Build history of the part. All positions in model axes, mm. Round coordinates to 2 decimals unless told otherwise and drop trailing zeros. Loops run counter-clockwise (first coordinate to the right, second up) from the corner with the lowest first, then second, coordinate; pieces in that order, holes last.
from build123d import *

# Parameters (mm, degrees)
EXTRUDE1_DEPTH = 25


with BuildPart() as part:
    # Sketch1 → Extrude1 (new body, symmetric)
    with BuildSketch(Plane.XY):
        with BuildLine():
            Line((0, -3), (0, -53.784988575))
            Line((0, -53.784988575), (0, -108))
            ThreePointArc((0, -108), (1.951109669, -110.810663458), (5.266552715, -109.96538515))
            ThreePointArc((5.266552715, -109.96538515), (8.33076313, -107.102662764), (11.924538917, -104.941797077))
            Line((11.924538917, -104.941797077), (78.267854785, -74.00540082))
            ThreePointArc((78.267854785, -74.00540082), (79.819077862, -72.312537889), (79.718923361, -70.018622673))
            Line((79.718923361, -70.018622673), (77.733454722, -65.760771437))
            ThreePointArc((77.733454722, -65.760771437), (76.399777201, -64.367593723), (74.493586828, -64.074202964))
            Line((74.493586828, -64.074202964), (49.961112633, -68.399940068))
            ThreePointArc((49.961112633, -68.399940068), (35.016620352, -65.086825893), (26.791994019, -52.176748561))
            Line((26.791994019, -52.176748561), (22.477002989, -27.705218377))
            ThreePointArc((22.477002989, -27.705218377), (21.821246743, -25.05746196), (20.811309078, -22.523560578))
            Line((20.811309078, -22.523560578), (10.816867263, -1.701806797))
            ThreePointArc((10.816867263, -1.701806797), (9.710018402, -0.460848606), (8.11229809, 0))
            Line((8.11229809, 0), (3, 0))
            ThreePointArc((3, 0), (0.878679656, -0.878679656), (0, -3))
        make_face()
    extrude(amount=EXTRUDE1_DEPTH, both=True)


solid = part.part
(1) Slice it at A-A on z = 13. List the corners of the cut face in (x, y), plus the area to 3 significant figures.
Responses:
outline: (0, -108) arc R3 ccw to (5.27, -109.97) arc R20 cw to (11.92, -104.94) - (78.27, -74.01) arc R3 ccw to (79.72, -70.02) - (77.73, -65.76) arc R3 ccw to (74.49, -64.07) - (49.96, -68.4) arc R20 cw to (26.79, -52.18) - (22.48, -27.71) arc R20 ccw to (20.81, -22.52) - (10.82, -1.7) arc R3 ccw to (8.11, 0) - (3, 0) arc R3 ccw to (0, -3) - close
area: 3,520 mm2
(2) Pull direction X, two halves, no side cores. Call faces 1 (the face through (78.74, -67.92, 0.35)), 2 (the face through (62.399, -66.207, 0.35)), 3 (the face through (0, -55, 0)): +X half, -X half, draft (parallel to the pull), parting line (faces both ways), or undercut.
Responses:
face 1: +X half
face 2: undercut
face 3: -X half
(3) Slice it at C-C on x = 43. List the corners of the cut face in (y, z), plus the area to 3 significant figures.
Responses:
outline: (-90.45, -25) - (-68.4, -25) - (-68.4, 25) - (-90.45, 25) - close
area: 1,100 mm2
(4) Probe line 1 (Y direction, x = 75.5, z = -19); line 2 (Y direction, x = 12, z = -4.5); line 3 (X direction, y = -100.5, z = -8). List the from-to ranges inside material, lowest first.
Responses:
line 1: y = -75.3 to -64.07
line 2: y = -104.91 to -4.17
line 3: x = 0 to 21.45
(5) Pin check, flat tips, straight feed: P1, Ø10, axis at y = -85, z = 1, coming from the +X side; P2, Ø4, axis at x = 32.5, z = -1, coming from the +Y side; P3, Ø5, axis at y = -67.5, z = 10.5, coming from the +X side; P4, Ø10, axis at x = 61, y = -92.5, coming from the -Z side. Stop position of each tip, or through.
Responses:
P1: stops at x = 65.41
P2: stops at y = -60.72
P3: stops at x = 79.71
P4: passes through
(6) Slice it at B-B on y = -19. List the corners of the cut face in (x, z).
Responses:
outline: (0, -25) - (19.12, -25) - (19.12, 25) - (0, 25) - close
